Source: CAD feature listing. Evaluate the final solid. Frame: model axes, mm. A direction names the side the tool comes from. Coordinates: 2 decimals unless noted, no trailing zeros. Order: outer loops, then holes, each group sorted by start corner. A loop starts at its lowest first (then second) coordinate and runs counter-clockwise, first axis right, second up.
```python
from build123d import *

# Parameters (mm, degrees)
SKETCH1_R           = 45
BOSS_EXTRUDE1_DEPTH = 5
SKETCH2_R           = 36.175
BOSS_EXTRUDE2_DEPTH = 5
SKETCH4_R           = 1.5
CUT_EXTRUDE2_DEPTH  = 66.383484153


with BuildPart() as part:
    # Sketch1 → Boss-Extrude1 (new, symmetric)
    with BuildSketch(Plane.XY):
        Circle(SKETCH1_R)
    extrude(amount=BOSS_EXTRUDE1_DEPTH, both=True)

    # Sketch2 → Boss-Extrude2 (add, symmetric)
    with BuildSketch(Plane.XY.offset(5)):
        Circle(SKETCH2_R)
    extrude(amount=BOSS_EXTRUDE2_DEPTH, both=True)

    # Sketch4 → Cut-Extrude2 (cut, through all)
    with BuildSketch(Plane(origin=(0, 0, -5), x_dir=(-1, 0, 0), z_dir=(0, 0, -1))):
        with Locations((-42, 0)):
            Circle(SKETCH4_R)
        with Locations((-21, 36.373066959)):
            Circle(SKETCH4_R)
        with Locations((21, 36.373066959)):
            Circle(SKETCH4_R)
        with Locations((42, 0)):
            Circle(SKETCH4_R)
        with Locations((21, -36.373066959)):
            Circle(SKETCH4_R)
        with Locations((-21, -36.373066959)):
            Circle(SKETCH4_R)
    extrude(amount=-CUT_EXTRUDE2_DEPTH, mode=Mode.SUBTRACT)


solid = part.part
```
1. Section query D-D, the plane z = -3. Output: boundary loops of the cut face in (x, y).
2. Material intervals for line 1 along Y through (x, z) = (21, -2.75); line 2 along Z through (x, y) = (-39, -2.5); line 3 along Y through (x, z) = (7.5, 5.25), sorted ascending.
3. Contact query for flat-ended pins moving along their axis: P1, Ø3.5, axis at x = 42, y = 0, coming from the -Z side; P2, Ø4, axis at x = 21, y = -36.37, coming from the +Z side; P3, Ø1, axis at y = 20, z = 8, coming from the -X side; P4, Ø5, axis at x = -25, z = 5, coming from the -Y side. Output: stop coordinate, or through.
4. Section query A-A, the plane y = 0. Output: boundary loops of the cut face in (x, z) (3 decimals).
5. Section query C-C, the plane x = 0. Output: boundary loops of the cut face in (y, z) (3 decimals).
6. Access query for faces 4 (the flat face through (-37, 0, 5)), 5 (the cylindrical face through (-19.81, -37.286, -0.07)). Directions: +Z, -Z, +X, -X, +Y, -Y. A direction counts if a zero-diameter tool reaches every point of the face in a straight line with its end or side. Return the directions, or none.
7. Draft query along X for faces 1 (the cylindrical face through (34.505, 10.866, 7.535)), 2 (the cylindrical face through (-20.8, 37.86, -0.07)), 3 (the flat face through (-1, 1, 10)). Return one class per face: +X half, -X half, draft (parallel to the pull), parting line (faces both ways), or undercut.
8. Section query B-B, the plane x = 21. Output: boundary loops of the cut face in (y, z).
Answer key:
1. outline: circle Ø90 at (0, 0); hole circle Ø3 at (-42, 0); hole circle Ø3 at (-21, -36.37); hole circle Ø3 at (-21, 36.37); hole circle Ø3 at (21, -36.37); hole circle Ø3 at (21, 36.37); hole circle Ø3 at (42, 0)
2. line 1: y = -39.8 to -37.87, -34.87 to 34.87, 37.87 to 39.8
2. line 2: z = -5 to 5
2. line 3: y = -35.39 to 35.39
3. P1: stops at z = -5
3. P2: stops at z = 5
3. P3: stops at x = -30.47
3. P4: stops at y = -38.97
4. outline: (-45, -5) - (-43.5, -5) - (-43.5, 5) - (-45, 5) - close; (-40.5, -5) - (40.5, -5) - (40.5, 5) - (36.175, 5) - (36.175, 10) - (-36.175, 10) - (-36.175, 5) - (-40.5, 5) - close; (43.5, -5) - (45, -5) - (45, 5) - (43.5, 5) - close
5. outline: (-45, -5) - (45, -5) - (45, 5) - (36.175, 5) - (36.175, 10) - (-36.175, 10) - (-36.175, 5) - (-45, 5) - close
6. face 4: +Z
6. face 5: +Z, -Z
7. face 1: parting line
7. face 2: undercut
7. face 3: draft
8. outline: (-39.8, -5) - (-37.87, -5) - (-37.87, 5) - (-39.8, 5) - close; (-34.87, -5) - (34.87, -5) - (34.87, 5) - (29.46, 5) - (29.46, 10) - (-29.46, 10) - (-29.46, 5) - (-34.87, 5) - close; (37.87, -5) - (39.8, -5) - (39.8, 5) - (37.87, 5) - close
